Geometry check sheet. Reference: drawing and pictorial views, mm from the part's lowest x, y, z. A direction names the side the tool comes from. Give positions to 0.01 mm unless a question says otherwise; leave off trailing zeros. Loops run counter-clockwise (first coordinate to the right, second up) from the corner with the lowest first, then second, coordinate; pieces in that order, holes last. Notation, with made-up numbers: (75.5, 87.25) -> (88.5, 87.25) arc R19 ccw to (88.5, 111.25) -> close; hole circle Ø1 at (-25, 9). An arc over 180 degrees is marked (long way). One line per item, written item: value. Start each with the question number.
(1) Tool access check on the marked faces 1, 2 and 3. Record the directions out of +Z, -Z, +X, -X, +Y, -Y that give a thin tool (end or side, any length) a straight path to the whole face; none if there is none.
(2) Sectioned sample at B-B, the plane y = 23.5. Record the cut outline in (x, z), then the cut area to 3 significant figures.
(3) Scan lines: line 1 along Y through (x, z) = (143, 8.5); line 2 along X through (y, z) = (9, 5.75). Record each from-to range of solid material in increasing order. Write a range as from..to.
(4) Sectioned sample at A-A, the plane z = 4. Record the cut outline in (x, y), then the cut area to 3 significant figures.
(5) Gauge pin test, flat ends, axial feed: pin 1 Ø5 at (x, z) = (3.5, 3.5) entering from -Y; pin 2 Ø3 at (y, z) = (23, 5.5) entering from +X; pin 3 Ø3 at (y, z) = (46.5, 3.5) entering from -X. Record the tip position at first contact, or that the pin passes through.
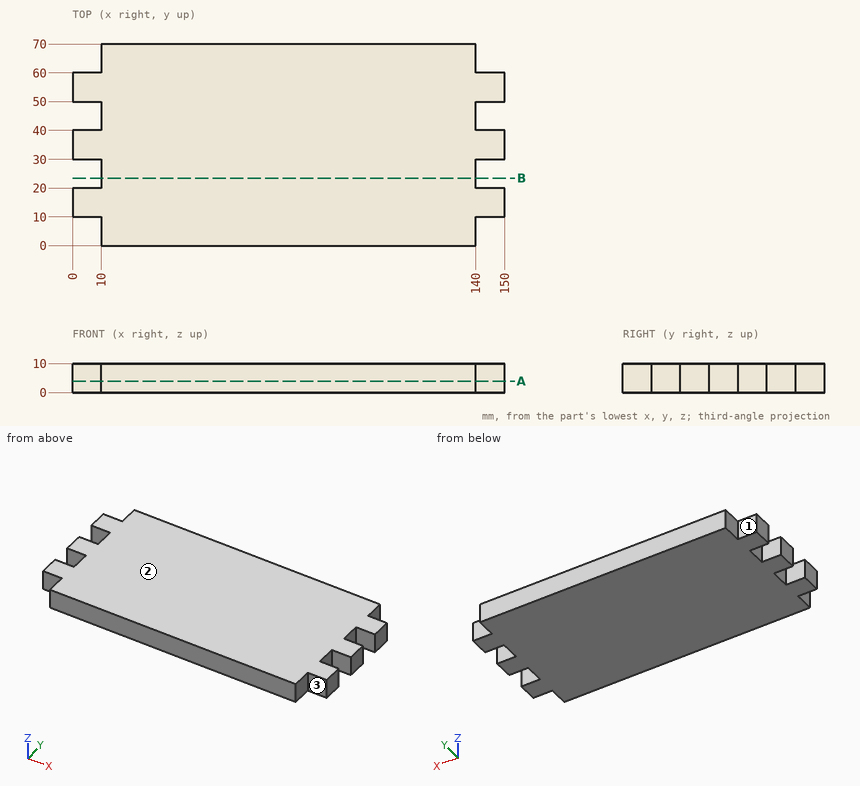
Calculated:
1. face 1: +Z, -Z, -X, +Y
1. face 2: +Z, +X, -X, +Y, -Y
1. face 3: +Z, -Z, +X, -Y
2. outline: (10, 0) -> (140, 0) -> (140, 10) -> (10, 10) -> close
2. area: 1,300 mm2
3. line 1: y = 10..20, 30..40, 50..60
3. line 2: x = 10..140
4. outline: (0, 10) -> (10, 10) -> (10, 0) -> (140, 0) -> (140, 10) -> (150, 10) -> (150, 20) -> (140, 20) -> (140, 30) -> (150, 30) -> (150, 40) -> (140, 40) -> (140, 50) -> (150, 50) -> (150, 60) -> (140, 60) -> (140, 70) -> (10, 70) -> (10, 60) -> (0, 60) -> (0, 50) -> (10, 50) -> (10, 40) -> (0, 40) -> (0, 30) -> (10, 30) -> (10, 20) -> (0, 20) -> close
4. area: 9,700 mm2
5. pin 1: stops at y = 10
5. pin 2: stops at x = 140
5. pin 3: stops at x = 10
